Can you work these out from the model? Positions are in its coordinate system, mm. Face numbers are marked on the shaded views. Coordinates: 2 decimals unless noted, no trailing zeros. Loops run counter-clockwise (first coordinate to the right, second up) from the corner with the lowest first, then second, coordinate; pieces in that order, holes last. Notation, with made-up numbers: (-31.5, -2.75) -> (13.5, -2.75) arc R28 cw to (13.5, 36.25) -> close; hole circle Ø5 at (-16.75, -24). An arc over 180 degrees is marked (long way). Put each result on its own line as item: value. Start each with the question number.
Item 1: If we section it at A-A on z = 176: Please give me the cut outline in (x, y).
Item 2: If we section it at B-B on y = 114: Please give me the cut outline in (x, z).
Item 3: We'd pull the mould along X, two halves only. Please class the marked faces 1, 2 and 3: pulls with the +X half, pulls with the -X half, needs draft (parallel to the pull), parting line crosses it, or undercut.
Item 4: If we section it at C-C on x = 172: Please give me the cut outline in (y, z), plus the area to 3 significant figures.
Item 5: Will these pins go through, and if not, where does the flat tip stop? P1, Ø12, axis at x = 58, y = -247.5, coming from the +Z side; P2, Ø0.5, axis at y = 238.5, z = 205.5, coming from the -X side; P3, Ø1.3, axis at x = -250, y = 237.5, coming from the +Z side.
Item 6: Please list where these lines run through material, in increasing order: L1, parallel to X at y = 234.5, z = 70.5; L2, parallel to Y at x = 193, z = 143; L3, parallel to Z at x = 82.5, y = -173.5. Write a range as from..to.
```python
from build123d import *

# Parameters (mm, degrees)
CROQUIS1_W              = 500
CROQUIS1_H              = 700
SALIENTE_EXTRUIR1_DEPTH = 200
VACIADO1_T              = -1
CROQUIS2_W              = 15
CROQUIS2_H              = 20
SALIENTE_EXTRUIR2_DEPTH = 2
SALIENTE_EXTRUIR3_START = -20
CROQUIS3_R              = 3
SALIENTE_EXTRUIR3_DEPTH = 20
SALIENTE_EXTRUIR4_START = -20
SALIENTE_EXTRUIR4_DEPTH = 20
CROQUIS5_W              = 42
CROQUIS5_H              = 60
CORTAR_EXTRUIR1_DEPTH   = 10
CROQUIS6_R              = 1.5
CORTAR_EXTRUIR2_DEPTH   = 10
CORTAR_EXTRUIR3_DEPTH   = 10
CROQUIS8_R              = 1.7
CORTAR_EXTRUIR4_DEPTH   = 10
CROQUIS9_R              = 24.815
CROQUIS9_R_2            = 1.85
CORTAR_EXTRUIR5_DEPTH   = 10


with BuildPart() as part:
    # Croquis1 → Saliente-Extruir1 (new body)
    with BuildSketch(Plane.XY):
        Rectangle(CROQUIS1_W, CROQUIS1_H)
    extrude(amount=SALIENTE_EXTRUIR1_DEPTH)

    # Vaciado1
    vaciado1_openings = [part.faces().sort_by_distance(p)[0] for p in [
        (0, 0, 200),
    ]]
    offset(amount=VACIADO1_T, openings=vaciado1_openings, kind=Kind.INTERSECTION)

    # Croquis2 → Saliente-Extruir2 (add)
    with BuildSketch(Plane(origin=(-249, 0, 0), x_dir=(0, 0, -1), z_dir=(1, 0, 0))):
        with Locations((-192.5, 240)):
            Rectangle(CROQUIS2_W, CROQUIS2_H)
        with Locations((-192.5, -240)):
            Rectangle(CROQUIS2_W, CROQUIS2_H)
    extrude(amount=SALIENTE_EXTRUIR2_DEPTH)

    # Croquis3 → Saliente-Extruir3 (add)
    with BuildSketch(Plane.XZ.offset(250).offset(SALIENTE_EXTRUIR3_START)):
        with Locations((-248.5, 202.5)):
            Circle(CROQUIS3_R)
    extrude(amount=SALIENTE_EXTRUIR3_DEPTH)

    # Croquis4 → Saliente-Extruir4 (add)
    with BuildSketch(Plane.XZ.offset(-230).offset(SALIENTE_EXTRUIR4_START)):
        with BuildLine():
            Line((-250, 199.901923789), (-247, 199.901923789))
            ThreePointArc((-247, 199.901923789), (-248.5, 205.5), (-250, 199.901923789))
        make_face()
    extrude(amount=SALIENTE_EXTRUIR4_DEPTH)

    # Croquis5 → Cortar-Extruir1 (cut)
    with BuildSketch(Plane(origin=(-249, 0, 0), x_dir=(0, 0, -1), z_dir=(1, 0, 0))):
        with Locations((-100, -150)):
            Rectangle(CROQUIS5_W, CROQUIS5_H)
    extrude(amount=-CORTAR_EXTRUIR1_DEPTH, mode=Mode.SUBTRACT)

    # Croquis6 → Cortar-Extruir2 (cut)
    with BuildSketch(Plane(origin=(-249, 0, 0), x_dir=(0, 0, -1), z_dir=(1, 0, 0))):
        with Locations((-118.05, -116.5)):
            Circle(CROQUIS6_R)
        with Locations((-82.05, -116.5)):
            Circle(CROQUIS6_R)
        with Locations((-82.05, -183.5)):
            Circle(CROQUIS6_R)
        with Locations((-118.05, -183.5)):
            Circle(CROQUIS6_R)
        Polygon((-204.984566909, 349), (-205.984152301, 348), (-703.777677317, 348), (-703.777677317, -350), (-205.984152301, -350), (-204.984566909, -351), (-204.984566909, -231), (-219.978347783, -231), (-219.978347783, -211), (-204.984566909, -211), (-204.984566909, 209), (-219.978347783, 209), (-219.978347783, 229), (-204.984566909, 229), align=None)
    extrude(amount=-CORTAR_EXTRUIR2_DEPTH, mode=Mode.SUBTRACT)

    # Croquis7 → Cortar-Extruir3 (cut)
    with BuildSketch(Plane(origin=(250, 0, 0), x_dir=(0, 0, -1), z_dir=(1, 0, 0))):
        with BuildLine():
            Line((-37.394449056, -342.885415535), (-57.394449056, -342.885415535))
            ThreePointArc((-57.394449056, -342.885415535), (-60.929982962, -341.420949441), (-62.394449056, -337.885415535))
            Line((-62.394449056, -337.885415535), (-62.394449056, -325.885415535))
            ThreePointArc((-62.394449056, -325.885415535), (-60.929982962, -322.349881629), (-57.394449056, -320.885415535))
            Line((-57.394449056, -320.885415535), (-37.394449056, -320.885415535))
            ThreePointArc((-37.394449056, -320.885415535), (-33.85891515, -322.349881629), (-32.394449056, -325.885415535))
            Line((-32.394449056, -325.885415535), (-32.394449056, -337.885415535))
            ThreePointArc((-32.394449056, -337.885415535), (-33.85891515, -341.420949441), (-37.394449056, -342.885415535))
        make_face()
    extrude(amount=-CORTAR_EXTRUIR3_DEPTH, mode=Mode.SUBTRACT)

    # Croquis8 → Cortar-Extruir4 (cut)
    with BuildSketch(Plane.ZY.offset(-249)):
        with Locations((27.394449056, -331.885415535)):
            Circle(CROQUIS8_R)
        with Locations((67.394449056, -331.885415535)):
            Circle(CROQUIS8_R)
    extrude(amount=-CORTAR_EXTRUIR4_DEPTH, mode=Mode.SUBTRACT)

    # Croquis9 → Cortar-Extruir5 (cut)
    with BuildSketch(Plane.XZ.offset(-349)):
        with Locations(Location((-129.140668179, 99.383298184, 0), (0, 0, 270))):
            Circle(CROQUIS9_R)
        with Locations(Location((-150.140668179, 120.423298184, 0), (0, 0, 270))):
            Circle(CROQUIS9_R_2)
        with Locations(Location((-108.140668179, 120.423298184, 0), (0, 0, 270))):
            Circle(CROQUIS9_R_2)
        with Locations(Location((-150.140668179, 78.423298184, 0), (0, 0, 270))):
            Circle(CROQUIS9_R_2)
        with Locations(Location((-108.140668179, 78.423298184, 0), (0, 0, 270))):
            Circle(CROQUIS9_R_2)
    extrude(amount=-CORTAR_EXTRUIR5_DEPTH, mode=Mode.SUBTRACT)


solid = part.part
```
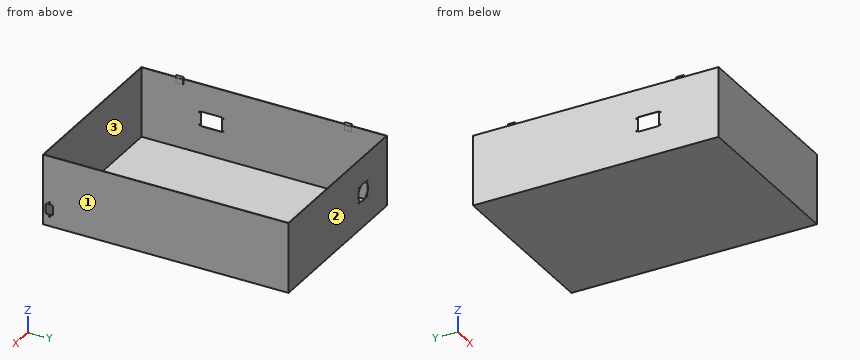
Solutions:
1. outline: (-250, -350) -> (250, -350) -> (250, 350) -> (-250, 350) -> close; hole (-249, -349) -> (249, -349) -> (249, 349) -> (-249, 349) -> close
2. outline: (-250, 0) -> (250, 0) -> (250, 200) -> (249, 200) -> (249, 1) -> (-249, 1) -> (-249, 200) -> (-250, 200) -> close
3. face 1: pulls with the +X half
3. face 2: needs draft
3. face 3: undercut
4. outline: (-350, 0) -> (350, 0) -> (350, 200) -> (349, 200) -> (349, 1) -> (-349, 1) -> (-349, 200) -> (-350, 200) -> close
4. area: 1,100 mm^2
5. P1: z = 1
5. P2: x = -249
5. P3: z = 204.98
6. L1: -250..-249, 249..250
6. L2: -350..-349, 349..350
6. L3: 0..1
